```python
from build123d import *

# Parameters (mm, degrees)
SKETCH1_R                 = 0.5
SKETCH1_R_2               = 5
BOSS_EXTRUDE1_DEPTH       = 5
SKETCH3_R                 = 1.3
BOSS_EXTRUDE4_DEPTH       = 5.7
BOSS_EXTRUDE6_DEPTH       = 1
FILLET1_R                 = 2.5
FILLET2_R                 = 2
F_2_0MM_DOWEL_HOLE1_D     = 2
F_2_0MM_DOWEL_HOLE1_DEPTH = 42.93
F_2_0MM_DOWEL_HOLE1_TIP   = 0.600860619


with BuildPart() as part:
    # Sketch1 → Boss-Extrude1 (new body)
    with BuildSketch(Plane(origin=(0, 0, 0), x_dir=(1, 0, 0), z_dir=(0, 1, 0))):
        with BuildLine():
            Line((1.767766953, 14.961194078), (14.961194078, 1.767766953))
            ThreePointArc((14.961194078, 1.767766953), (15.693427125, 0), (14.961194078, -1.767766953))
            Line((14.961194078, -1.767766953), (1.767766953, -14.961194078))
            ThreePointArc((1.767766953, -14.961194078), (0, -15.693427125), (-1.767766953, -14.961194078))
            Line((-1.767766953, -14.961194078), (-14.961194078, -1.767766953))
            ThreePointArc((-14.961194078, -1.767766953), (-15.693427125, 0), (-14.961194078, 1.767766953))
            Line((-14.961194078, 1.767766953), (-1.767766953, 14.961194078))
            ThreePointArc((-1.767766953, 14.961194078), (0, 15.693427125), (1.767766953, 14.961194078))
        make_face()
        with Locations(Location((0, 10.365, 0), (0, 0, 270))):
            Circle(SKETCH1_R, mode=Mode.SUBTRACT)
        with Locations(Location((0, -10.365, 0), (0, 0, 270))):
            Circle(SKETCH1_R, mode=Mode.SUBTRACT)
        with Locations(Location((10.365, 0, 0), (0, 0, 270))):
            Circle(SKETCH1_R, mode=Mode.SUBTRACT)
        with Locations(Location((-10.365, 0, 0), (0, 0, 270))):
            Circle(SKETCH1_R, mode=Mode.SUBTRACT)
        with Locations(Location((0, 0, 0), (0, 0, 270))):
            Circle(SKETCH1_R_2, mode=Mode.SUBTRACT)
    extrude(amount=BOSS_EXTRUDE1_DEPTH)

    # Sketch3 → Boss-Extrude4 (add)
    # profile 1 of 4: a face of its own
    with BuildSketch(Plane(origin=(0, -2.7, 0), x_dir=(1, 0, 0), z_dir=(0, 1, 0))):
        Polygon((-4.949747468, -10.537489101), (-0.637994164, -14.849242405), (-4.949747468, -19.160995709), (-9.261500772, -14.849242405), align=None)
        with Locations(Location((-4.949747468, -14.849242405, 0), (0, 0, 90))):
            Circle(SKETCH3_R, mode=Mode.SUBTRACT)
    # profile 2 of 4: a face of its own
    with BuildSketch(Plane(origin=(0, -2.7, 0), x_dir=(1, 0, 0), z_dir=(0, 1, 0))):
        Polygon((-6.717514421, -8.769722148), (-11.029267725, -13.081475452), (-9.261500772, -14.849242405), (-4.949747468, -10.537489101), align=None)
    # profile 3 of 4: a face of its own
    with BuildSketch(Plane(origin=(0, -2.7, 0), x_dir=(1, 0, 0), z_dir=(0, 1, 0))):
        Polygon((19.160995709, 4.949747468), (14.849242405, 9.261500772), (10.537489101, 4.949747468), (14.849242405, 0.637994164), align=None)
        with Locations(Location((14.849242405, 4.949747468, 0), (0, 0, 90))):
            Circle(SKETCH3_R, mode=Mode.SUBTRACT)
    # profile 4 of 4: a face of its own
    with BuildSketch(Plane(origin=(0, -2.7, 0), x_dir=(1, 0, 0), z_dir=(0, 1, 0))):
        Polygon((13.081475452, 11.029267725), (14.849242405, 9.261500772), (10.537489101, 4.949747468), (8.769722148, 6.717514421), align=None)
    extrude(amount=BOSS_EXTRUDE4_DEPTH)


with BuildPart() as boss_extrude6_tool:
    # Sketch7 → Boss-Extrude6 (new, symmetric)
    with BuildSketch(Plane(origin=(2.707626069, -2.13e-07, 2.707626069), x_dir=(0.7071067811865474, 0, -0.7071067811865478), z_dir=(0.7071067811865467, -5.5755039757469385e-08, 0.7071067811865462))):
        Polygon((11.829161787, 5.00000052), (17.04887, 3.00000056), (11.829161787, 3.00000052), align=None)
        Polygon((-11.829161787, 5.00000052), (-17.04887, 3.00000056), (-11.829161787, 3.00000052), align=None)
    extrude(amount=BOSS_EXTRUDE6_DEPTH, both=True)


with BuildPart() as part_1:
    add(part.part)


with BuildPart() as part_2:
    # Boss-Extrude6: joined with boss_extrude6_tool
    add(part_1.part.fuse(boss_extrude6_tool.part, tol=0.00001))

    # Fillet1
    fillet1_edges = [part_2.edges().sort_by_distance(p)[0] for p in [
        (-7.338376652, 1.5, 9.390584379),
        (-1.184018869, 1.5, 15.395267109),
        (9.390584379, 1.5, -7.338376652),
        (15.395267109, 1.5, -1.184018869),
    ]]
    fillet(fillet1_edges, radius=FILLET1_R)

    # Fillet2
    # the kernel refuses this fillet: 2 mm, written as the material it takes off along each edge
    with BuildSketch(Plane(origin=(-4.949747468, -7.7, 19.160995709), x_dir=(-0.7071067811865471, 0, -0.707106781186548), z_dir=(0, 1, 0)), Plane(origin=(13.081475452, -7.7, -11.029267725), x_dir=(0.7071067811865476, 0, 0.7071067811865476), z_dir=(0, 1, 0))) as fillet2_piece_1:
        with BuildLine():
            CenterArc((FILLET2_R, -FILLET2_R), FILLET2_R, 90, 90)
            Line((0, -FILLET2_R), (0, 0))
            Line((0, 0), (FILLET2_R, 0))
        make_face()
    extrude(amount=15.7, mode=Mode.SUBTRACT)
    with BuildSketch(Plane(origin=(-11.029267725, -7.7, 13.081475452), x_dir=(0.707106781186547, 0, 0.7071067811865479), z_dir=(0, 1, 0)), Plane(origin=(19.160995709, -7.7, -4.949747468), x_dir=(-0.7071067811865482, 0, -0.7071067811865469), z_dir=(0, 1, 0))) as fillet2_piece_2:
        with BuildLine():
            CenterArc((FILLET2_R, FILLET2_R), FILLET2_R, 180, 90)
            Line((0, FILLET2_R), (0, 0))
            Line((0, 0), (FILLET2_R, 0))
        make_face()
    extrude(amount=15.7, mode=Mode.SUBTRACT)

    # Ø2.0mm Dowel Hole1
    with Locations(Plane.XZ):
        with Locations((0, 10.365), (10.365, 0), (-10.365, 0), (0, -10.365)):
            Hole(F_2_0MM_DOWEL_HOLE1_D / 2, depth=F_2_0MM_DOWEL_HOLE1_DEPTH)
            with Locations((0, 0, -(F_2_0MM_DOWEL_HOLE1_DEPTH + F_2_0MM_DOWEL_HOLE1_TIP / 2))):  # 118° drill point
                Cone(0, F_2_0MM_DOWEL_HOLE1_D / 2, F_2_0MM_DOWEL_HOLE1_TIP, mode=Mode.SUBTRACT)


solid = part_2.part
```
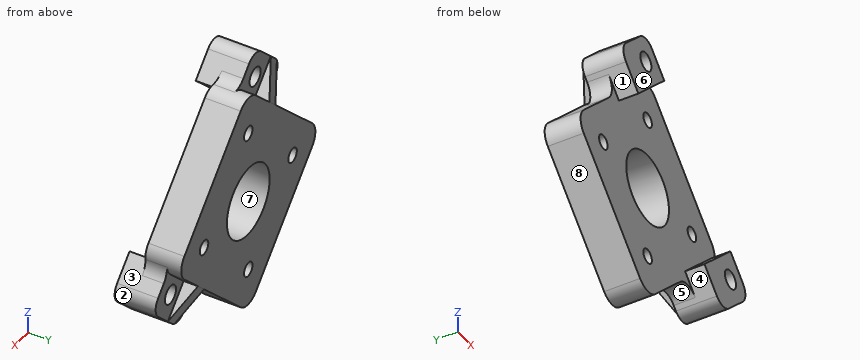
CAD build for the part. Positions are in the model's coordinates, mm. Face numbers are marked on the shaded views. A direction names the side the tool comes from. Round coordinates to 2 decimals unless told otherwise and drop trailing zeros. Order: outer loops, then holes, each group sorted by start corner. A loop starts at its lowest first (then second) coordinate and runs counter-clockwise, first axis right, second up.
Item 1: Mould opens along X. For the marked faces 6, 7 and 8 say: pulls with the +X half, pulls with the -X half, needs draft (parallel to the pull), parting line crosses it, or undercut.
Item 2: Tool access for the marked faces 1, 2, 3, 4 and 5: list every direction of +Z, -Z, +X, -X, +Y, -Y with a clear straight run to the whole face (end or side of a thin tool).
Item 3: Saw through at C-C on y = 1.5. State how many separate pieces and enclosed holes the cut face has, then the cut area to 3 significant figures.
Item 4: Saw through at D-D on z = -12. Write the cut outline in (x, y).
Item 5: Probe line 1 along Y through (x, z) = (4.5, -11); line 2 along X through (y, z) = (3.75, 0.5); line 3 along X through (y, z) = (2.5, 10). List the from-to ranges inside material, lowest first.
Item 6: Saw through at B-B on z = 2.5. Write the cut outline in (x, y), then the cut area to 3 significant figures.
Item 7: Saw through at A-A on x = 0.5. Write the cut outline in (y, z).
Item 8: Pin check, flat tips, straight feed: pin 1 (2.5 mm diameter, centred on x = 0, z = -10.365, fed in from -Y); pin 2 (1.2 mm diameter, centred on x = 11.5, z = -8.5, fed in from +Y); pin 3 (3 mm diameter, centred on x = -1.5, y = 1.5, fed in from +Z). Stop position of each tip, or through.
Reported:
1. face 6: needs draft
1. face 7: undercut
1. face 8: pulls with the -X half
2. face 1: -X, -Y
2. face 2: +X, +Y, -Y
2. face 3: +Z, +X, -Y
2. face 4: -Z, -Y
2. face 5: -Z, +Y, -Y
3. separate pieces: 1
3. enclosed holes: 7
3. area: 542 mm2
4. outline: (-4.73, 0) - (4.73, 0) - (4.73, 5) - (-4.73, 5) - close
5. line 1: y = 0 to 5
5. line 2: x = -15.64 to -11.23, -9.5 to -4.97, 4.97 to 9.5, 11.23 to 15.64
5. line 3: x = -8.45 to -0.93, 0.93 to 6.73
6. outline: (-14.23, 0) - (-4.33, 0) - (-4.33, 5) - (-14.23, 5) - close; (4.33, 0) - (14.23, 0) - (14.23, 5) - (4.33, 5) - close
6. area: 99.0 mm2
7. outline: (0, -15.64) - (5, -15.64) - (5, -11.23) - (0, -11.23) - close; (0, -9.5) - (5, -9.5) - (5, -4.97) - (0, -4.97) - close; (0, 4.97) - (5, 4.97) - (5, 9.5) - (0, 9.5) - close; (0, 11.23) - (5, 11.23) - (5, 15.64) - (0, 15.64) - close
8. pin 1: stops at y = 0
8. pin 2: stops at y = 3
8. pin 3: stops at z = 17.21
